The drawing under review shows one solid part. Ordinate dimensions are in mm from its lowest x, y, z. A direction names the side the tool comes from. Give positions to 0.01 mm unless a question says otherwise; leave off trailing zeros. Write each loop counter-clockwise with the first axis right and the second up, starting at its lowest first coordinate (ties: lowest second). Pieces come first, ordered by that corner, then holes.
Q1. We need section C-C (y = 93). Write out the cut boundary in (x, z).
Q2. Mouldability with a two-part tool opening along Y and no side actions: class the marked faces 3, 4 and 5 as released by +Y, released by -Y, zero draft, split by the parting line, or undercut.
Q3. We need section A-A (y = 75). Write out the cut boundary in (x, z).
Q4. Machinability: for the marked faces 1 and 2, which of the approach directions +Z, -Z, +X, -X, +Y, -Y give a long, thin tool a straight path to every point of the face, cutting with its end or side? Answer none if there is none.
Q5. Insertion check: P1, Ø4, axis at y = 35, z = 9, coming from the -X side; P2, Ø10, axis at x = 135, y = 75, coming from the +Z side. Each pin has a flat end and moves straight along its axis. Give the tip position at first contact, or say it passes through.
Q6. For line 1 (X direction, y = 75, z = 10.5); line 2 (X direction, y = 89, z = 27.25); line 3 (X direction, y = 74, z = 27), list the stretches that pass through material, from the lowest coordinate up.
Q7. We need section D-D (x = 135). Write out the cut boundary in (y, z).
Q8. We need section B-B (z = 18.25). Write out the cut boundary in (x, y), then the cut area to 3 significant figures.
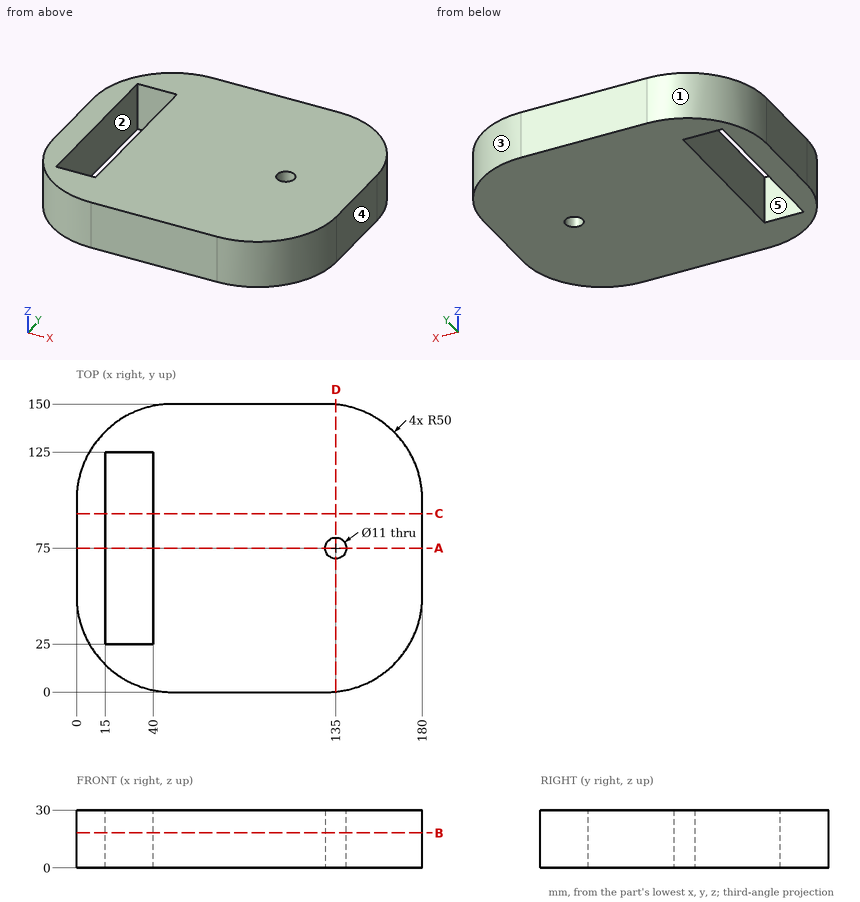
Computed:
1. outline: (0, 0) - (15, 0) - (15, 30) - (0, 30) - close; (40, 0) - (180, 0) - (180, 30) - (40, 30) - close
2. face 3: released by +Y
2. face 4: zero draft
2. face 5: undercut
3. outline: (0, 0) - (15, 0) - (15, 30) - (0, 30) - close; (40, 0) - (129.5, 0) - (129.5, 30) - (40, 30) - close; (140.5, 0) - (180, 0) - (180, 30) - (140.5, 30) - close
4. face 1: +Z, -Z, -X, +Y
4. face 2: +Z, -Z
5. P1: stops at x = 1.72
5. P2: passes through
6. line 1: x = 0 to 15, 40 to 129.5, 140.5 to 180
6. line 2: x = 0 to 15, 40 to 180
6. line 3: x = 0 to 15, 40 to 129.59, 140.41 to 180
7. outline: (0.25, 0) - (69.5, 0) - (69.5, 30) - (0.25, 30) - close; (80.5, 0) - (149.75, 0) - (149.75, 30) - (80.5, 30) - close
8. outline: (0, 50) arc R50 ccw to (50, 0) - (130, 0) arc R50 ccw to (180, 50) - (180, 100) arc R50 ccw to (130, 150) - (50, 150) arc R50 ccw to (0, 100) - close; hole (15, 25) - (40, 25) - (40, 125) - (15, 125) - close; hole circle Ø11 at (135, 75)
8. area: 22,300 mm2
